Model file for the job. Use its own axes, mm. A direction names the side the tool comes from. Coordinates: 2 decimals unless noted, no trailing zeros. Write each loop counter-clockwise with the first axis right and the second up, starting at its lowest first coordinate (ties: lowest second). Pieces come first, ordered by that corner, then holes. Notation, with made-up numbers: M 73,36.5 L 111,36.5 A23 ccw 111,57.5 Z; hole C 52,7 d7. An arc over 180 degrees is marked long. Answer in a Markdown table with one row per item. Add a question column.
```python
from build123d import *

# Parameters (mm, degrees)
F1_DEPTH = 12
F2_T     = -2


with BuildPart() as f1:
    # F0 (on Front) → F1 (new body)
    with BuildSketch(Plane.XZ):
        with BuildLine():
            Line((0, 87.2677220979), (-18.6475409836, 62.2677220979))
            ThreePointArc((-18.6475409836, 62.2677220979), (1.1915533371, -64.9890775488), (16.3524590164, 62.909435573))
            Line((16.3524590164, 62.909435573), (0, 87.2677220979))
        make_face()
    extrude(amount=F1_DEPTH)

    # F2
    f2_openings = [f1.faces().sort_by_distance(p)[0] for p in [
        (-0.019386, -12, 1.977046),
    ]]
    offset(amount=F2_T, openings=f2_openings, kind=Kind.INTERSECTION)


solid = f1.part
```
1) Slice it at C-C (x = 32). Give the cut face in (y, z).
2) Slice it at B-B (z = 0). Give the cut face in (x, y), then the cut area to 3 significant figures.
3) Which spindle directions (+Z, -Z, +X, -X, +Y, -Y) get a long thin tool onto all of the face, cutting with end or side? Do faces 4 (the face through (-8.64, -6.93, 72.34)), 5 (the face through (-1.419, -5.916, -64.985)). Say none if no direction does.
4) Two-plate mould, pull along X, no slides. Class faces 1 (the face through (-53.3, -12, 34)), 2 (the face through (-1, -2, -5)), 3 (the face through (-9.193, -5.916, 74.943)): released by +X, released by -X, zero draft, split by the parting line, or undercut.
5) Flat gauge pins, fed straight in: pin 1 Ø12 at (x, z) = (39, 17) entering from -Y; pin 2 Ø6 at (x, y) = (-40.5, -6.5) entering from -Z; pin 3 Ø4 at (x, y) = (31.5, -10) entering from -Z. Where does each tip first touch, or does it go through?
6) Slice it at A-A (y = -6.25). Give the cut face in (x, z).
7) Drill centre lines: probe 1 along X at (y, z) = (-5.75, 0); probe 2 along Y at (x, z) = (55, 7); probe 3 along Z at (x, y) = (0, -9.5). Where is each one in solid material? Low to high.
Ans:
| question | item | result |
|---|---|---|
| 1 | outline | M -12,-56.58 L 0,-56.58 L 0,56.58 L -12,56.58 L -12,54.27 L -2,54.27 L -2,-54.27 L -12,-54.27 Z |
| 2 | outline | M -65,-12 L -63,-12 L -63,-2 L 63,-2 L 63,-12 L 65,-12 L 65,0 L -65,0 Z |
| 2 | area | 300 mm2 |
| 3 | face 4 | -Y |
| 3 | face 5 | +Y, -Y |
| 4 | face 1 | zero draft |
| 4 | face 2 | undercut |
| 4 | face 3 | released by -X |
| 5 | pin 1 | stops at y = -2 |
| 5 | pin 2 | stops at z = -53.09 |
| 5 | pin 3 | stops at z = -57.92 |
| 6 | outline | M -18.65,62.27 A65 ccw long 16.35,62.91 L 0,87.27 Z; hole M -17.44,60.54 A63 ccw long 15.12,61.16 L -0.09,83.81 Z |
| 7 | probe 1 | x = -65 to -63, 63 to 65 |
| 7 | probe 2 | y = -2 to 0 |
| 7 | probe 3 | z = -65 to -63, 83.68 to 87.27 |
